Autodesk Inventor part; units mm, degrees
ref_plane "YZ Plane" through (0, 0, 0) normal (1, 0, 0) x (0, 1, 0)
ref_plane "XZ Plane" through (0, 0, 0) normal (0, 1, 0) x (-1, 0, 0)
ref_plane "XY Plane" through (0, 0, 0) normal (0, 0, 1) x (1, 0, 0)
sketch "Sketch1" plane through (0, 0, 0) normal (0, 1, 0) x (-1, 0, 0)
  line L0 (-16.5, 16.5) -> (16.5, 16.5)
  line L1 (16.5, 16.5) -> (16.5, -16.5)
  line L2 (16.5, -16.5) -> (-16.5, -16.5)
  line L3 (-16.5, -16.5) -> (-16.5, 16.5)
  line L4 (-16.5, 16.5) -> (16.5, -16.5) construction
  line L5 (16.5, 16.5) -> (-16.5, -16.5) construction
  point P0 (0, 0)
  dimension "d0" = 33
  dimension "d1" = 33
extrude "Extrusion1" add sketch "Sketch1" along normal blind 62
sketch "Sketch2" plane through (0, 62, 0) normal (0, 1, 0) x (1, 0, 0)
  circle A0 centre (0, 0) radius 6
  dimension "d4" = 12
extrude "Extrusion2" add sketch "Sketch2" along normal blind 7
sketch "Sketch3" plane through (16.5, 0, 16.5) normal (1, 0, 0) x (0, 0, -1)
  circle A0 centre (8.5, 57) radius 1.575
  line L0 (-0.0785, 57) -> (33, 57)
  line L1 (33, 0) -> (33, 62)
  line L2 (0, 62) -> (33, 62)
  line L3 (33, 62) -> (0, 62)
  line L4 (16.5, 62) -> (16.5, 57)
  line L5 (0, 17) -> (33, 17)
  line L6 (16.5, 57) -> (16.5, 17)
  line L7 (16.5, 37) -> (33, 37)
  circle A1 centre (24.5, 57) radius 1.575
  circle A2 centre (8.5, 17) radius 1.575
  circle A3 centre (24.5, 17) radius 1.575
  point P0 (16.5, 0)
  dimension "d7" = 3.15
  dimension "d8" = 5
  dimension "d9" = 8
  dimension "d10" = 40
hole "Hole1" at (16.5, 57, 8) at (16.5, 57, -8) at (16.5, 17, 8) at (16.5, 17, -8) direction (-1, 0, 0) diameter 2.459 depth 10 tip angle 118
sketch "Sketch4" plane through (0, 0, 0) normal (0, -1, 0) x (1, 0, 0)
  circle A0 centre (0, 0) radius 16.5
  line L0 (16.5, -16.5) -> (-16.5, -16.5)
  line L1 (-16.5, 16.5) -> (16.5, 16.5)
  line L2 (16.5, 16.5) -> (16.5, -16.5)
  line L3 (16.5, -16.5) -> (-16.5, -16.5)
  line L4 (-16.5, -16.5) -> (-16.5, 16.5)
  line L5 (-16.5, 16.5) -> (16.5, -16.5) construction
  line L6 (16.5, 16.5) -> (-16.5, -16.5) construction
  dimension "d18" = 33
extrude "Extrusion3" cut sketch "Sketch4" against normal blind 11 contours L2 L0 A0 | A0 L1 L2 | A0 L4 L1 | L0 L4 A0
equation "\"d0\" = laser_y"
equation "\"d1\" = laser_z"
equation "\"d2\" = laser_x"
equation "\"d4\" = laser_diameter"
equation "\"d7\" = m3_diameter"
equation "\"d10\" = laser_screw_spacing_x"
equation "\"d18\" = laser_y"
equation "\"thick_acrylic\" = 5.88"
equation "\"thin_acrylic\" = 3.15"
equation "\"clear_acrylic\" = 3.15"
equation "\"wood_thickness\" = 6.72"
equation "\"al1_thickness\" = 1.5875"
equation "\"m3_diameter\" = 3.15"
equation "\"m4_diameter\" = 4.2"
equation "\"m5_diameter\" = 5.25"
equation "\"brass_insert_drill\" = 4"
equation "\"m5_brass_insert_drill\" = 6.7"
equation "\"m5_press_nut_drill\" = 6.35"
equation "\"m3_main_length\" = 14"
equation "\"m3_main_nut_width\" = 5.7"
equation "\"m3_main_nut_thickness\" = 2.5"
equation "\"m3_main_extra\" = 1"
equation "\"stepper_screw_space\" = 35"
equation "\"stepper_shaft_diameter\" = 5"
equation "\"stepper_body_diameter\" = 28"
equation "\"laser_body_diameter\" = 12"
equation "\"t_carrier\" = 6.72"
equation "\"t_wall\" = 5.88"
equation "\"t_window\" = 3.15"
equation "\"carrier_y\" = 181"
equation "\"carrier_z\" = 233.04"
equation "\"carrier_z2\" = 283.04"
equation "\"protection_slot\" = 30.2"
equation "\"protection_slot_offset\" = 37.75"
equation "\"protection_slot_length\" = 20.6"
equation "\"window_z\" = 185"
equation "\"window_y\" = 49.56"
equation "\"window_slot\" = 25"
equation "\"door_sensor\" = 35"
equation "\"reservoir_x\" = 151"
equation "\"reservoir_y\" = 151"
equation "\"linear_bearing_spacing\" = 207"
equation "\"linear_bearing_z\" = 304.8"
equation "\"threaded_rod_z\" = 203.2"
equation "\"motor_spacing\" = 287"
equation "\"t_tray\" = 3.15"
equation "\"tray_border\" = 15"
equation "\"tray_x\" = 151"
equation "\"tray_y\" = 181"
equation "\"bed_t\" = 1.5875"
equation "\"bed_y2\" = 45.96"
equation "\"bed_fold_x\" = 15"
equation "\"bed_gap\" = 0.3"
equation "\"t_inner_tray\" = 5.88"
equation "\"t_tape\" = 3"
equation "\"inner_tray_x\" = 145"
equation "\"inner_tray_y\" = 145"
equation "\"inner_tray_border\" = 5"
equation "\"inner_tray_radius\" = 24"
equation "\"t_bottom_clear\" = 3.15"
equation "\"bottom_clear_border\" = 5"
equation "\"brass_keep_out\" = 8"
equation "\"tape_keep_out\" = 2"
equation "\"tape_thickness\" = 2"
equation "\"t_crane\" = 6.72"
equation "\"crane_x\" = 244.56"
equation "\"end_stop_offset_x\" = 83"
equation "\"end_stop_spacing\" = 19"
equation "\"thumb_nut_offset_y\" = 11.72"
equation "\"thumb_nut_diameter\" = 7"
equation "\"z_min_from_center\" = 72.28"
equation "\"t_frame\" = 6.72"
equation "\"frame_top_z\" = 295"
equation "\"frame_bottom_z\" = 225"
equation "\"frame_y\" = 68.44"
equation "\"frame_border\" = 39.5"
equation "\"frame_foot_z\" = 49.5"
equation "\"frame_foot_extension\" = 6"
equation "\"frame_tilt\" = 0"
equation "\"printer_z\" = 289"
equation "\"lcd_x\" = 72"
equation "\"lcd_y\" = 25"
equation "\"subframe_y_offset\" = 27.5"
equation "\"laser_y_offset\" = 19.4"
equation "\"laser_diameter\" = 12"
equation "\"laser_y\" = 33"
equation "\"laser_z\" = 33"
equation "\"laser_x\" = 62"
equation "\"laser_screw_spacing_x\" = 40"
equation "\"laser_screw_spacing_y\" = 16"
equation "\"t_galvo_frame\" = 6.72"
equation "\"galvo_frame_x\" = 66"
equation "\"galvo_frame_z\" = 65"
equation "\"galvo_frame_y_offset\" = 27.5"
equation "\"drawer_x\" = 181"
equation "\"drawer_y\" = 49.56"
equation "\"drawer_z\" = 206.72"
equation "\"drawer_z_from_bottom\" = 25"
equation "\"drawer_foot_mount\" = 18"
equation "\"asym_key\" = 0"
equation "\"small_round\" = 2"
properties part number "laser"
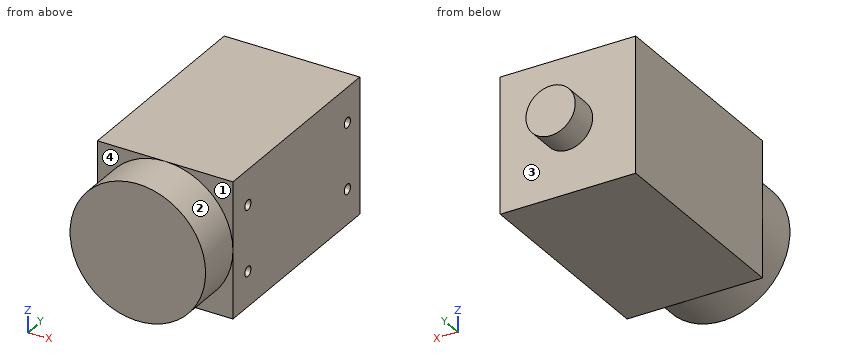
Source: CAD feature listing. Evaluate the final solid. Frame: model axes, mm. Face numbers are marked on the shaded views. A direction names the side the tool comes from. Coordinates: 2 decimals unless noted, no trailing zeros. Loops run counter-clockwise (first coordinate to the right, second up) from the corner with the lowest first, then second, coordinate; pieces in that order, holes last. Notation, with made-up numbers: (51.5, 80.25) - (72.5, 80.25) arc R25 cw to (72.5, 101.25) - close; hole circle Ø4 at (-30.75, 11). An arc over 180 degrees is marked (long way). Answer as CSV lines item,"result".
1. Section B-B (x = 4). Return loops of the section in (y, z).
Established:
outline,"(0, -16.01) - (11, -16.01) - (11, -16.5) - (62, -16.5) - (62, -4.47) - (69, -4.47) - (69, 4.47) - (62, 4.47) - (62, 16.5) - (11, 16.5) - (11, 16.01) - (0, 16.01) - close"
2. Section C-C (z = 11.5). Return loops of the section in (x, y), then the cut area to 3 significant figures.
Established:
outline,"(-16.5, 11) - (-11.83, 11) - (-11.83, 0) - (11.83, 0) - (11.83, 11) - (16.5, 11) - (16.5, 62) - (-16.5, 62) - close"
area,"1,940 mm2"
3. Ray query, line 1 (Y direction, x = 13, z = 8); line 2 (Z direction, x = 14, y = 17); line 3 (Y direction, x = 9.5, z = 7). Return the intervals inside material, ascending.
Established:
line 1,"y = 0 to 15.77, 18.23 to 55.77, 58.23 to 62"
line 2,"z = -16.5 to -9.23, -6.77 to 6.77, 9.23 to 16.5"
line 3,"y = 0 to 16.28, 17.72 to 56.28, 57.72 to 62"
4. Contact query for flat-ended pins moving along their axis: pin 1 (2 mm diameter, centred on y = 17, z = 8, fed in from +X); pin 2 (5 mm diameter, centred on x = -9, z = -9, fed in from -Y). Output: stop coordinate, or through.
Established:
pin 1,"stops at x = 6.36"
pin 2,"stops at y = 0"
5. Reachability of the marked faces 1, 2, 3 and 4 from +Z, -Z, +X, -X, +Y, -Y: full face, straight path, thin tool, end or side. Return the list, or none.
Established:
face 1,"+Z, +X, -Y"
face 2,"-Y"
face 3,"+Y"
face 4,"+Z, -X, -Y"
6. Section A-A (x = 13.5). Return loops of the section in (y, z).
Established:
outline,"(0, -9.49) - (11, -9.49) - (11, -16.5) - (62, -16.5) - (62, 16.5) - (11, 16.5) - (11, 9.49) - (0, 9.49) - close; hole circle Ø2.46 at (17, -8); hole circle Ø2.46 at (17, 8); hole circle Ø2.46 at (57, -8); hole circle Ø2.46 at (57, 8)"
7. Section D-D (x = -9). Return loops of the section in (y, z).
Established:
outline,"(0, -13.83) - (11, -13.83) - (11, -16.5) - (62, -16.5) - (62, 16.5) - (11, 16.5) - (11, 13.83) - (0, 13.83) - close"
